Could you check a few things on this model? Use its own coordinates, in mm. A direction names the side the tool comes from. Give positions to 0.01 mm unless a question says otherwise; leave off trailing zeros. Loops run counter-clockwise (first coordinate to the right, second up) from the corner with the lowest first, then second, coordinate; pieces in that order, holes last.
1. For P1, Ø6, axis at x = 31.53, y = 25, coming from the +Z side; P2, Ø7, axis at x = 378.5, z = 4.5, coming from the -Y side; P3, Ø1, axis at y = -22.5, z = 6.5, coming from the -X side; P4, Ø11.5, axis at x = 334.53, y = 25, coming from the +Z side, each with a flat end and sliding along its axis, tell me the tip position at first contact or that it passes through.
2. For faces 1 (the flat face through (308.032, -30, 7)), 2 (the flat face through (360.032, 30, 7)), 3 (the flat face through (181, 20, 7)), 4 (the flat face through (-25, -20, 7)), 5 (the flat face through (6.032, 30, 7)), which set-ups out of +Z, -Z, +X, -X, +Y, -Y let a thin tool reach every point of the face, with its end or its side?
3. Thinking about a two-plate mould opening in X: for faces 6 (the flat face through (58.032, -30, 7)), 7 (the flat face through (423.032, 0, 7)), 8 (the flat face through (-56.968, 0, 7)), which applies, +X half, -X half, draft (parallel to the pull), parting line (faces both ways), or undercut?
4. I need wall thicknesses on line 1 along X through (y, z) = (21, 12); line 2 along Y through (x, z) = (149.5, 1.75); line 3 along Y through (x, z) = (30, 5). Which ranges of each line are inside material? Lowest first, please.
5. Imagine slicing it at A-A (z = 9.25). List the corners of the cut face in (x, y) for me, plus the area to 3 significant figures.
6. Imagine slicing it at B-B (x = 185). List the corners of the cut face in (y, z) for me.
```python
from build123d import *

# Parameters (mm, degrees)
BOSS_EXTRUDE1_DEPTH = 14
SKETCH3_R           = 3.65
CUT_EXTRUDE1_DEPTH  = 14


with BuildPart() as part:
    # Sketch2 → Boss-Extrude1 (new body)
    with BuildSketch(Plane.XY):
        Polygon((-56.968136793, -20), (-56.968136793, 20), (6.031863207, 20), (6.031863207, 40), (58.031863207, 40), (58.031863207, 20), (308.031863207, 20), (308.031863207, 40), (360.031863207, 40), (360.031863207, 20), (423.031863207, 20), (423.031863207, -20), (360.031863207, -20), (360.031863207, -40), (308.031863207, -40), (308.031863207, -20), (58.031863207, -20), (58.031863207, -40), (6.031863207, -40), (6.031863207, -20), align=None)
    extrude(amount=BOSS_EXTRUDE1_DEPTH)

    # Sketch3 → Cut-Extrude1 (cut)
    with BuildSketch(Plane.XY.offset(14)):
        with Locations((31.531863207, 25)):
            Circle(SKETCH3_R)
        with Locations(Location((31.531863207, -25, 0), (0, 0, 180))):
            Circle(SKETCH3_R)
        with Locations((334.531863207, -25)):
            Circle(SKETCH3_R)
        with Locations(Location((334.531863207, 25, 0), (0, 0, 180))):
            Circle(SKETCH3_R)
    extrude(amount=-CUT_EXTRUDE1_DEPTH, mode=Mode.SUBTRACT)


solid = part.part
```
Derived:
1. P1: passes through
1. P2: stops at y = -20
1. P3: stops at x = 6.03
1. P4: stops at z = 14
2. face 1: +Z, -Z, -Y
2. face 2: +Z, -Z, +X, +Y
2. face 3: +Z, -Z, +Y
2. face 4: +Z, -Z, -X, -Y
2. face 5: +Z, -Z, -X, +Y
3. face 6: undercut
3. face 7: +X half
3. face 8: -X half
4. line 1: x = 6.03 to 58.03, 308.03 to 360.03
4. line 2: y = -20 to 20
4. line 3: y = -40 to -28.31, -21.69 to 21.69, 28.31 to 40
5. outline: (-56.97, -20) - (6.03, -20) - (6.03, -40) - (58.03, -40) - (58.03, -20) - (308.03, -20) - (308.03, -40) - (360.03, -40) - (360.03, -20) - (423.03, -20) - (423.03, 20) - (360.03, 20) - (360.03, 40) - (308.03, 40) - (308.03, 20) - (58.03, 20) - (58.03, 40) - (6.03, 40) - (6.03, 20) - (-56.97, 20) - close; hole circle Ø7.3 at (31.53, -25); hole circle Ø7.3 at (31.53, 25); hole circle Ø7.3 at (334.53, -25); hole circle Ø7.3 at (334.53, 25)
5. area: 23,200 mm2
6. outline: (-20, 0) - (20, 0) - (20, 14) - (-20, 14) - close
